Autodesk Inventor part; units mm, degrees
ref_plane "Work Plane4" through (-1.75, 0, 0) normal (1, 0, 0) x (0, 1, 0)
ref_plane "XZ Plane" through (0, 0, 0) normal (0, 1, 0) x (-1, 0, 0)
ref_plane "XY Plane" through (0, 0, 0) normal (0, 0, 1) x (1, 0, 0)
sketch "Sketch4" plane through (0, 0, 0) normal (0, 1, 0) x (-1, 0, 0)
  line L0 (21.5786, 9.75) -> (-18.7214, 9.75)
  line L1 (-18.7214, 9.75) -> (-18.7214, -9.75)
  line L2 (-18.7214, -9.75) -> (21.5786, -9.75)
  line L3 (21.5786, -9.75) -> (21.5786, 9.75)
  point P0 (0, 0)
  point P1 (21.5786, 0)
  dimension "d6" = 19.5
  dimension "d7" = 40.3
extrude "Extrusion2" add sketch "Sketch4" along normal blind 35.5
sketch "Sketch5" plane through (0, 35.5, 0) normal (0, 1, 0) x (1, 0, 0)
  point P0 (0, 0)
sketch "Sketch6" plane through (0, 35.5, 0) normal (0, 1, 0) x (1, 0, 0)
  point P0 (0, 0)
sketch "Sketch7" plane through (0, 35.5, 0) normal (0, 1, 0) x (1, 0, 0)
  point P0 (0, 0)
sketch "Sketch9" plane through (0, 35.5, 0) normal (0, 1, 0) x (1, 0, 0)
  circle A0 centre (-11.7806, 0) radius 9.75
  line L0 (18.7214, 9.75) -> (-21.5786, 9.75)
  point P0 (0, 0)
extrude "Extrusion3" add sketch "Sketch9" along normal blind 2
sketch "Sketch12" plane through (0, 35.5, 0) normal (0, 1, 0) x (1, 0, 0)
  arc A0 (-11.7806, -9.75) -> (-11.7806, 9.75) centre (-11.7806, 0) ccw
  arc A1 (-9.1237, -9.381) -> (-9.0416, 9.3574) centre (-11.7806, 0) ccw
  line L0 (-9.1237, -9.381) -> (12.6403, -9.381)
  line L1 (12.6403, -9.381) -> (12.6403, 9.3574)
  line L2 (12.6403, 9.3574) -> (-9.0416, 9.3574)
  point P0 (0, 0)
extrude "Extrusion4" add sketch "Sketch12" along normal blind 2
sketch "Sketch13" plane through (0, 35.5, 0) normal (0, 1, 0) x (1, 0, 0)
  line L0 (-21.5786, 9.75) -> (-21.5786, -9.75) construction
  line L1 (-21.5786, 0) -> (18, 0) construction
  line L2 (12.6403, -9.381) -> (12.6403, 9.3574)
  arc A0 (12.6403, -6) -> (15.5036, 0) centre (8.5831, -0.3807) ccw
  arc A1 (15.5036, 0) -> (12.6403, 6) centre (8.5831, 0.3807) ccw
  line L3 (12.6403, -6) -> (12.6403, 6)
  line L4 (12.6403, 9.3574) -> (12.6403, -9.381)
  point P0 (0, 0)
extrude "Extrusion5" add sketch "Sketch13" along normal blind 1.8
sketch "Sketch14" plane through (0, 37.5, 0) normal (0, 1, 0) x (1, 0, 0)
  arc A0 (-9.0416, 9.3574) -> (-9.1237, -9.381) centre (-11.7806, 0) ccw
  circle A1 centre (-11.7806, 0) radius 6.395
  point P0 (0, 0)
  dimension "d16" = 12.79
extrude "Extrusion6" add sketch "Sketch14" along normal blind 1.2
sketch "Sketch16" plane through (-11.7806, 38.7, 0) normal (0, 1, 0) x (1, 0, 0)
  circle A0 centre (0, 0) radius 6.395
  circle A1 centre (0, 0) radius 5.6569
  point P0 (11.7806, 0)
extrude "Extrusion7" add sketch "Sketch16" along normal blind 0.6 contours A1
sketch "Sketch17" plane through (-11.7806, 39.3, 0) normal (0, 1, 0) x (1, 0, 0)
  circle A0 centre (0, 0) radius 6.395
  circle A1 centre (0, 0) radius 2.85
  point P0 (11.7806, 0)
  dimension "d21" = 5.7
extrude "Extrusion8" add sketch "Sketch17" along normal blind 3 contours A1
sketch "Sketch18" plane through (-11.7806, 42.3, 0) normal (0, 1, 0) x (1, 0, 0)
  circle A0 centre (0, 0) radius 2.85
  circle A1 centre (0, 0) radius 1.4142
  point P0 (11.7806, 0)
extrude "Extrusion9" cut sketch "Sketch18" against normal blind 3 contours A1
sketch "Sketch19" plane through (-21.5786, 0, -9.75) normal (-1, 0, 0) x (0, 0, 1)
  line L0 (0, 35.5) -> (0, 30.5) construction
  line L1 (19.5, 0) -> (19.5, 35.5)
  line L2 (0, 30.5) -> (19.5, 30.5)
  line L3 (19.5, 30.5) -> (19.5, 29)
  line L4 (19.5, 29) -> (0, 29)
  line L5 (0, 29) -> (0, 30.5)
  point P0 (9.75, 0)
  dimension "d26" = 5
extrude "Extrusion10" add sketch "Sketch19" along normal blind 5.8
sketch "Sketch20" plane through (-21.5786, 30.5, 9.75) normal (0, 1, 0) x (1, 0, 0)
  point P0 (21.5786, 9.75)
sketch "Sketch22" plane through (-21.5786, 30.5, 9.75) normal (0, 1, 0) x (1, 0, 0)
  circle A0 centre (-3.8003, 4.6866) radius 2.25
  line L0 (-11.4938, 9.75) -> (0.0481, 9.75) construction
  arc A1 (9.7981, 19.5) -> (9.7981, 0) centre (9.7981, 9.75) ccw construction
  circle A2 centre (-3.8003, 14.8134) radius 2.25
  point P0 (21.5786, 9.75)
  dimension "d29" = 4.5
hole "Hole1" at (-25.3789, 30.5, 5.0634) at (-25.3789, 30.5, -5.0634) direction (0, -1, 0) diameter 4.5 depth 8 tip angle 118
fillet "Fillet1" radius 1 1 edges at (-27.3786, 29.75, 9.75)
fillet "Fillet2" radius 1 1 edges at (-27.3786, 29.75, -9.75)
fillet "Fillet3" radius 1 4 edges at (-21.5786, 33, 9.75) (-21.5786, 33, -9.75) (18.7214, 17.75, 9.75) (18.7214, 17.75, -9.75)
fillet "Fillet4" radius 1 2 edges at (-21.5786, 14.5, 9.75) (-21.5786, 14.5, -9.75)
ref_plane "Work Plane4" through (-1.75, 0, 0) normal (1, 0, 0) x (0, 1, 0)
mirror "Mirror2" about plane through (-1.75, 0, 0) normal (1, 0, 0) of "Extrusion10", "Hole1", "Fillet1", "Fillet2"
fillet "Fillet5" radius 1 8 edges at (-1.4286, 0, 9.75) (18.4285, 0, 9.4571) (18.7214, 0, 0) (18.4285, 0, -9.4571) (-1.4286, 0, -9.75) (-21.2858, 0, -9.4571) (-21.5786, 0, 0) (-21.2858, 0, 9.4571)
sketch "Sketch26" plane through (0, 35.5, 0) normal (0, 1, 0) x (1, 0, 0)
  point P0 (0, 0)
properties part number "servo"
Geometry check sheet. Reference: the model listing, model coordinates, mm. A direction names the side the tool comes from. Give positions to 0.01 mm unless a question says otherwise; leave off trailing zeros. Loops run counter-clockwise (first coordinate to the right, second up) from the corner with the lowest first, then second, coordinate; pieces in that order, holes last.
(1) Section check A-A on y = 32. Record the cut outline in (x, z).
From the geometry:
outline: (-21.58, -8.75) arc R1 ccw to (-20.58, -9.75) - (17.72, -9.75) arc R1 ccw to (18.72, -8.75) - (18.72, 8.75) arc R1 ccw to (17.72, 9.75) - (-20.58, 9.75) arc R1 ccw to (-21.58, 8.75) - close
(2) Thickness scan on L1, parallel to X at y = 41.3, z = 0; L2, parallel to X at y = 28.5, z = 6; L3, parallel to Y at x = -7, z = -6.5. Record the ranges inside material, lowest first.
From the geometry:
L1: x = -14.63 to -13.19, -10.37 to -8.93
L2: x = -21.58 to 18.72
L3: y = 0 to 37.5
(3) Section check C-C on x = 1.5. Record the cut outline in (y, z).
From the geometry:
outline: (0, -8.75) arc R1 ccw to (1, -9.75) - (35.5, -9.75) - (35.5, -9.36) - (37.5, -9.36) - (37.5, 9.38) - (35.5, 9.38) - (35.5, 9.75) - (1, 9.75) arc R1 ccw to (0, 8.75) - close
(4) Section check B-B on x = 16.5. Record the cut outline in (y, z).
From the geometry:
outline: (0, -8.75) arc R1 ccw to (1, -9.75) - (35.5, -9.75) - (35.5, 9.75) - (1, 9.75) arc R1 ccw to (0, 8.75) - close
(5) Depth check by flat-ended pin: pin 1 Ø7 at (x, z) = (-25.38, 5.06) entering from +Y; pin 2 Ø0.6 at (y, z) = (36, -4) entering from +X; pin 3 Ø3 at (x, z) = (-14.5, 4.5) entering from +Y. Enter the tip coordinate at first touch or a pass-through.
From the geometry:
pin 1: stops at y = 30.5
pin 2: stops at x = 14.67
pin 3: stops at y = 39.3
(6) Set-up check for faces 5 (the cylindrical face through (-9.148, 40.779, -1.092)), 6 (the flat face through (18.721, 15, 0)), 7 (the flat face through (18.721, 33, 0)), 8 (the flat face through (-21.579, 33, 0)): record each of +Z, -Z, +X, -X, +Y, -Y from which the full face is reachable in a straight line by a thin tool's end or side.
From the geometry:
face 5: +Y
face 6: +Z, -Z, +X, -Y
face 7: +Z, -Z, +X, +Y
face 8: +Z, -Z, -X, +Y
(7) Release check for a two-part mould opening along Z. For faces 1 (the cylindrical face through (-23.13, 29.74, -5.15)), 2 (the flat face through (12.64, 36.5, 6.4)), 3 (the flat face through (-4, 18, -9.75)), 4 (the cylindrical face through (-5.68, 38.09, 1.92)) record: released by +Z, released by -Z, zero draft, split by the parting line, or undercut.
From the geometry:
face 1: undercut
face 2: zero draft
face 3: released by -Z
face 4: split by the parting line
